Can you work these out from the model? Positions are in its coordinate system, mm. Coordinates: 2 decimals unless noted, no trailing zeros. Write each loop counter-clockwise with the first axis right and the second up, starting at its lowest first coordinate (ties: lowest second). Pieces come first, ordered by that corner, then holes. Notation, with made-up numbers: (51, -29) -> (56, -29) arc R21 cw to (56, -12) -> close; hole circle Ø11 at (39.25, 22). An arc over 180 degrees is marked (long way). Answer as CSV lines item,"result". Start each with the question number.
```python
from build123d import *

# Parameters (mm, degrees)
F0_R     = 3
F0_R_2   = 4
F1_DEPTH = 2.5


with BuildPart() as f1:
    # F0 (on Right) → F1 (new body)
    with BuildSketch(Plane.YZ):
        with BuildLine():
            Line((-23.98203, 3.693869), (-46.064754, -3.255427))
            ThreePointArc((-46.064754, -3.255427), (-51.363547, -13.05589), (-41.727933, -18.648851))
            Line((-41.727933, -18.648851), (1.935375, -7.762366))
            ThreePointArc((1.935375, -7.762366), (6.502157, -4.660681), (7.972699, 0.660358))
            Line((7.972699, 0.660358), (4.232059, 45.822225))
            ThreePointArc((4.232059, 45.822225), (4.149011, 48.51186), (4.344404, 51.195673))
            Line((4.344404, 51.195673), (9.922664, 95.788309))
            ThreePointArc((9.922664, 95.788309), (2.127756, 106.800584), (-9.540323, 100.02661))
            Line((-9.540323, 100.02661), (-24.498515, 52.410936))
            ThreePointArc((-24.498515, 52.410936), (-25.05208, 49.583636), (-24.969341, 46.703842))
            Line((-24.969341, 46.703842), (-19.841616, 10.252983))
            ThreePointArc((-19.841616, 10.252983), (-20.709418, 6.214413), (-23.98203, 3.693869))
        make_face()
        with Locations((-43.663308, -10.886485)):
            Circle(F0_R, mode=Mode.SUBTRACT)
        Circle(F0_R, mode=Mode.SUBTRACT)
        with Locations((-12.096095, 48.514786)):
            Circle(F0_R_2, mode=Mode.SUBTRACT)
        with Locations((-4.838438, 77.623658)):
            Circle(F0_R, mode=Mode.SUBTRACT)
        with Locations((0, 97.029573)):
            Circle(F0_R_2, mode=Mode.SUBTRACT)
    extrude(amount=F1_DEPTH)


solid = f1.part
```
Q1. Imagine slicing it at D-D (z = 40). Write out the boundary of the cut face in (x, y).
Q2. Imagine slicing it at C-C (z = -1.5). Write out the boundary of the cut face in (x, y), then the cut area to 3 significant figures.
Q3. Imagine slicing it at A-A (y = 0). Write out the boundary of the cut face in (x, z).
Q4. Imagine slicing it at B-B (x = 0.5). Write out the boundary of the cut face in (y, z).
Q5. For pin 1 (10 mm diameter, centred on y = -12.5, z = 87.5, fed in from -X); pin 2 (1 mm diameter, centred on x = 1, y = 1, fed in from +Z); pin 3 (1 mm diameter, centred on x = 2, z = 49, fed in from +Y), each with a flat end and sliding along its axis, tell me the tip position at first contact or that it passes through.
Q6. If we mould it in two halves opening along Y, with no side actions, what happens to faces 1 (the face through (1.23, 6.13, 22.93)), 2 (the face through (1, -3, 0)), 3 (the face through (1.23, -22.44, 28.73))? For each: released by +Y, released by -Y, zero draft, split by the parting line, or undercut.
Q7. I need wall thicknesses on L1, parallel to Z at x = 0.6, y = 0; L2, parallel to Y at x = 1.5, z = 53; L3, parallel to Z at x = 2.05, y = -8. Which ranges of each line are inside material? Lowest first, please.
Entries:
1,outline,"(0, -24.03) -> (2.5, -24.03) -> (2.5, 4.71) -> (0, 4.71) -> close"
2,outline,"(0, -40.49) -> (2.5, -40.49) -> (2.5, -2.6) -> (0, -2.6) -> close; (0, 2.6) -> (2.5, 2.6) -> (2.5, 7.86) -> (0, 7.86) -> close"
2,area,"108 mm2"
3,outline,"(0, -8.24) -> (2.5, -8.24) -> (2.5, -3) -> (0, -3) -> close; (0, 3) -> (2.5, 3) -> (2.5, 93.03) -> (0, 93.03) -> close; (0, 101.03) -> (2.5, 101.03) -> (2.5, 107.03) -> (0, 107.03) -> close"
4,outline,"(-46.06, -3.26) arc R8 ccw to (-41.73, -18.65) -> (1.94, -7.76) arc R8 ccw to (7.97, 0.66) -> (4.23, 45.82) arc R26 cw to (4.34, 51.2) -> (9.92, 95.79) arc R10 ccw to (-9.54, 100.03) -> (-24.5, 52.41) arc R13 ccw to (-24.97, 46.7) -> (-19.84, 10.25) arc R6 cw to (-23.98, 3.69) -> close; hole circle Ø6 at (-43.66, -10.89); hole circle Ø8 at (-12.1, 48.51); hole circle Ø6 at (-4.84, 77.62); hole circle Ø8 at (0, 97.03); hole circle Ø6 at (0, 0)"
5,pin 1,"x = 0"
5,pin 2,"z = 107.02"
5,pin 3,"y = 4.19"
6,face 1,"released by +Y"
6,face 2,"undercut"
6,face 3,"released by -Y"
7,L1,"-8.24 to -3, 3 to 93.03, 101.03 to 107.03"
7,L2,"-24.31 to 4.57"
7,L3,"-10.24 to 103.03"
